Design review of the part built by this model. Coordinates are the model's own, in mm. Round coordinates to 2 decimals unless told otherwise and drop trailing zeros. Loops run counter-clockwise (first coordinate to the right, second up) from the corner with the lowest first, then second, coordinate; pieces in that order, holes last. Notation, with made-up numbers: (86, -20.75) - (118, -20.75) arc R16 cw to (118, 10.25) - close; hole circle Ø11 at (9.5, -12.5). An arc over 180 degrees is marked (long way). Use one line per item in the form item = value. Start each with the question number.
(1) We need section B-B, the plane x = -124. Write out the cut boundary in (y, z), then the cut area to 3 significant figures.
(2) Wall thickness on probe 1 along Y at (x, z) = (-124.5, 32); probe 2 along X at (y, z) = (108, 39); probe 3 along Y at (x, z) = (-125, 55.5): over which ranges is each line inside the solid? List them lowest first. Write a range as [from, to].
(3) We need section A-A, the plane z = 23. Write out the cut boundary in (x, y), then the cut area to 3 significant figures.
from build123d import *

# Parameters (mm, degrees)
BOX002_W     = 42
BOX002_H     = 42
BOX002_DEPTH = 47
CHAMFER_SIZE = 4


with BuildPart() as nema:
    # Box002 → Box002 (new body)
    with BuildSketch(Plane(origin=(85, 69, 20), x_dir=(1, 0, 0), z_dir=(0, 0, 1))):
        with Locations((21, 21)):
            Rectangle(BOX002_W, BOX002_H)
    extrude(amount=BOX002_DEPTH)

    # Chamfer
    chamfer_edges = [nema.edges().sort_by_distance(p)[0] for p in [
        (85, 69, 43.5),
        (85, 111, 43.5),
        (127, 69, 43.5),
        (127, 111, 43.5),
    ]]
    chamfer(chamfer_edges, length=CHAMFER_SIZE)


with BuildPart() as nema001:
    # Part__Mirroring003: instance of NEMA
    add(nema.part.mirror(Plane(origin=(0, 0, 0), x_dir=(0, -1, 0), z_dir=(1, 0, 0))))


solid = nema001.part
Data:
q1.outline = (70, 20) - (110, 20) - (110, 67) - (70, 67) - close
q1.area = 1,880 mm^2
q2.probe_1 = [70.5, 109.5]
q2.probe_2 = [-126, -86]
q2.probe_3 = [71, 109]
q3.outline = (-127, 73) - (-123, 69) - (-89, 69) - (-85, 73) - (-85, 107) - (-89, 111) - (-123, 111) - (-127, 107) - close
q3.area = 1,730 mm^2
